```python
from build123d import *

# Parameters (mm, degrees)
CUT_EXTRUDE1_DEPTH = 1.65


with BuildPart() as part:
    # Sketch1 → Revolve1 (revolve)
    with BuildSketch(Plane.XY, mode=Mode.PRIVATE) as revolve1_sk:
        with BuildLine():
            Line((-1.462050681, 4.37208714), (0, 4.5))
            Line((0, 4.5), (0, 2.5))
            Line((0, 2.5), (3.641673123, 2.5))
            Line((3.641673123, 2.5), (3.641673123, 1.85))
            Line((3.641673123, 1.85), (8, 0))
            Line((8, 0), (-3.3, 0))
            ThreePointArc((-3.3, 0), (-3.190657425, 1.617218351), (-2.864619959, 3.205))
            ThreePointArc((-2.864619959, 3.205), (-2.346005844, 4.008071364), (-1.462050681, 4.37208714))
        make_face()
    revolve(revolve1_sk.sketch.rotate(Axis((-3.3, 0, 0), (1, 0, 0)), 180), axis=Axis((-3.3, 0, 0), (1, 0, 0)))

    # Sketch2 → Cut-Extrude1 (cut)
    with BuildSketch(Plane(origin=(-3.3, 0, 0), x_dir=(0, 0, -1), z_dir=(1, 0, 0))):
        with BuildLine():
            Line((0.6, 1.5), (0.6, 2.45))
            Line((0.6, 2.45), (-0.6, 2.45))
            Line((-0.6, 2.45), (-0.6, 1.5))
            ThreePointArc((-0.6, 1.5), (-0.863603897, 0.863603897), (-1.5, 0.6))
            Line((-1.5, 0.6), (-2.45, 0.6))
            Line((-2.45, 0.6), (-2.45, -0.6))
            Line((-2.45, -0.6), (-1.5, -0.6))
            ThreePointArc((-1.5, -0.6), (-0.863603897, -0.863603897), (-0.6, -1.5))
            Line((-0.6, -1.5), (-0.6, -2.45))
            Line((-0.6, -2.45), (0.6, -2.45))
            Line((0.6, -2.45), (0.6, -1.5))
            ThreePointArc((0.6, -1.5), (0.863603897, -0.863603897), (1.5, -0.6))
            Line((1.5, -0.6), (2.45, -0.6))
            Line((2.45, -0.6), (2.45, 0.6))
            Line((2.45, 0.6), (1.5, 0.6))
            ThreePointArc((1.5, 0.6), (0.863603897, 0.863603897), (0.6, 1.5))
        make_face()
    extrude(amount=CUT_EXTRUDE1_DEPTH, mode=Mode.SUBTRACT)


solid = part.part
```
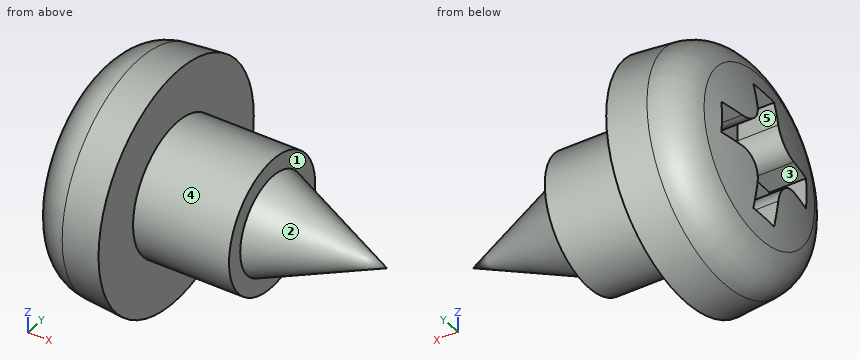
Geometry: final body of the model. Coordinates: model frame, mm. Face numbers are marked on the shaded views. A direction names the side the tool comes from. Round coordinates to 2 decimals unless told otherwise and drop trailing zeros. Order: outer loops, then holes, each group sorted by start corner. A loop starts at its lowest first (then second) coordinate and runs counter-clockwise, first axis right, second up. Notation, with made-up numbers: M 74.25,61.25 L 89.25,61.25 A18 ccw 89.25,85.25 Z; hole C -3,33 d10. An arc over 180 degrees is marked long. Use one line per item in the form item = value. Start each with the question number.
Q1. Mould query, pull axis Y, two halves, no side actions, for the marked faces 1, 2 and 3. Classes: +Y half, -Y half, draft (parallel to the pull), parting line (faces both ways), or undercut.
Q2. Pin query (flat end, axial travel): pin 1 Ø0.8 at (x, y) = (-2.5, 2) entering from +Z; pin 2 Ø0.8 at (x, y) = (-2.5, -2) entering from -Z; pin 3 Ø0.6 at (x, z) = (-2.5, 0) entering from +Y. Return the tip coordinate at first contact, or that it passes through.
Q3. Cut plane A-A (x = 1). Return loops of the section in (y, z).
Q4. Access query for the marked faces 4 and 5. Directions: +Z, -Z, +X, -X, +Y, -Y. A direction counts if a zero-diameter tool reaches every point of the face in a straight line with its end or side. Return the directions, or none.
Q5. Cut plane B-B (x = -0.25). Return loops of the section in (y, z), and give its area (3 significant figures).
Q6. Material intervals for line 1 (Y direction, x = 1.5, z = 2); line 2 (Y direction, x = 3.5, z = -0.5); line 3 (Y direction, x = -2, z = -1.5), sorted ascending. Write a range as [from, to].
Geometry results:
q1.face_1 = draft
q1.face_2 = parting line
q1.face_3 = undercut
q2.pin_1 = 3.74
q2.pin_2 = -3.74
q2.pin_3 = 4.12
q3.outline = C 0,0 d5
q4.face_4 = +X
q4.face_5 = -X
q5.outline = C 0,0 d8.96
q5.area = 63.0 mm^2
q6.line_1 = [-1.5, 1.5]
q6.line_2 = [-2.45, 2.45]
q6.line_3 = [-3.95, -0.6], [0.6, 3.95]
